```python
from build123d import *

# Parameters (mm, degrees)
SKETCH1_R           = 38.3
SKETCH1_R_2         = 3.1
SKETCH1_R_3         = 21
BOSS_EXTRUDE1_DEPTH = 4
CUT_EXTRUDE1_DEPTH  = 10


with BuildPart() as part:
    # Sketch1 → Boss-Extrude1 (new body)
    with BuildSketch(Plane(origin=(0, 0, 0), x_dir=(1, 0, 0), z_dir=(0, 1, 0))):
        with Locations(Location((0, 0, 0), (0, 0, 270))):
            Circle(SKETCH1_R)
        with Locations(Location((30, 0, 0), (0, 0, 270))):
            Circle(SKETCH1_R_2, mode=Mode.SUBTRACT)
        with Locations(Location((0, 0, 0), (0, 0, 270))):
            Circle(SKETCH1_R_3, mode=Mode.SUBTRACT)
        with Locations(Location((15, -25.980762114, 0), (0, 0, 270))):
            Circle(SKETCH1_R_2, mode=Mode.SUBTRACT)
        with Locations(Location((-15, -25.980762114, 0), (0, 0, 270))):
            Circle(SKETCH1_R_2, mode=Mode.SUBTRACT)
        with Locations(Location((-30, 0, 0), (0, 0, 270))):
            Circle(SKETCH1_R_2, mode=Mode.SUBTRACT)
        with Locations(Location((-15, 25.980762114, 0), (0, 0, 270))):
            Circle(SKETCH1_R_2, mode=Mode.SUBTRACT)
        with Locations(Location((15, 25.980762114, 0), (0, 0, 270))):
            Circle(SKETCH1_R_2, mode=Mode.SUBTRACT)
    extrude(amount=BOSS_EXTRUDE1_DEPTH)

    # Sketch2 → Cut-Extrude1 (cut)
    with BuildSketch(Plane(origin=(0, 4, 0), x_dir=(1, 0, 0), z_dir=(0, 1, 0))):
        with BuildLine():
            Line((6, 50.276302336), (6, 14.297506921))
            ThreePointArc((6, 14.297506921), (13.428105902, 7.752720557), (15.382004204, -1.952601038))
            Line((15.382004204, -1.952601038), (46.540555031, -19.941998745))
            ThreePointArc((46.540555031, -19.941998745), (-43.84951462, -25.31652907), (6, 50.276302336))
        make_face()
    extrude(amount=-CUT_EXTRUDE1_DEPTH, mode=Mode.SUBTRACT)


solid = part.part
```
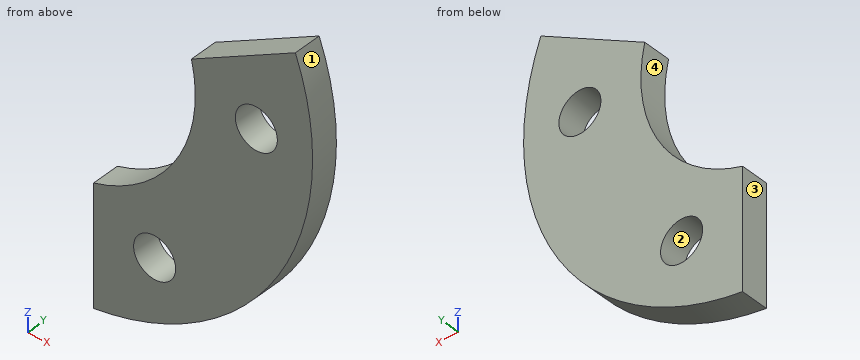
Check sheet for the modelled part. Datum: model origin and axes. Units: mm. Face numbers are marked on the shaded views. Coordinates: 2 decimals unless noted, no trailing zeros. Order: outer loops, then holes, each group sorted by start corner. A loop starts at its lowest first (then second) coordinate and runs counter-clockwise, first axis right, second up. Notation, with made-up numbers: (52.5, 22.5) -> (90.5, 22.5) arc R30 cw to (90.5, 50.5) -> close; hole circle Ø6 at (17.5, 71.25). An arc over 180 degrees is marked (long way). Write each question's results on one line, items separated by ' | '. Start each with the question number.
1) Section check C-C (y = 3.35). Enter the section's corners in (x, z).
2) Section check D-D (x = 35). Enter the section's corners in (y, z).
3) Depth check by flat-ended pin: pin 1 (2 mm diameter, centred on x = 12.5, y = 1, fed in from -Z); pin 2 (1 mm diameter, centred on y = 2.5, z = -6.5, fed in from +X). Enter the tip coordinate at first touch or a pass-through.
4) Section check B-B (x = 30). Enter the section's corners in (y, z), and give its area (3 significant figures).
5) Draft check along Z on the marked faces 1, 2, 3 and 4. Enter one of: pulls with the +Z half, pulls with the -Z half, needs draft (parallel to the pull), parting line crosses it, or undercut.
6) Material ranges on line 1 along X through (y, z) = (0.9, 0); line 2 along Z through (x, y) = (32, 2); line 3 along X through (y, z) = (2.55, -32), recorded low to high.
7) Section check A-A (z = 0). Enter the section's corners in (x, y).
Checked values:
1) outline: (6, -37.83) arc R38.3 ccw to (35.76, 13.72) -> (20.43, 4.87) arc R21 cw to (6, -20.12) -> close; hole circle Ø6.2 at (15, -25.98); hole circle Ø6.2 at (30, 0)
2) outline: (0, -15.55) -> (4, -15.55) -> (4, 13.28) -> (0, 13.28) -> close
3) pin 1: z = -36.53 | pin 2: x = 37.83
4) outline: (0, -23.81) -> (4, -23.81) -> (4, -3.1) -> (0, -3.1) -> close; (0, 3.1) -> (4, 3.1) -> (4, 10.39) -> (0, 10.39) -> close | area: 112 mm²
5) face 1: parting line crosses it | face 2: undercut | face 3: needs draft | face 4: undercut
6) line 1: 21 to 26.9, 33.1 to 38.3 | line 2: -21.04 to -2.37, 2.37 to 11.55 | line 3: 6 to 21.04
7) outline: (21, 0) -> (26.9, 0) -> (26.9, 4) -> (21, 4) -> close; (33.1, 0) -> (38.3, 0) -> (38.3, 4) -> (33.1, 4) -> close
